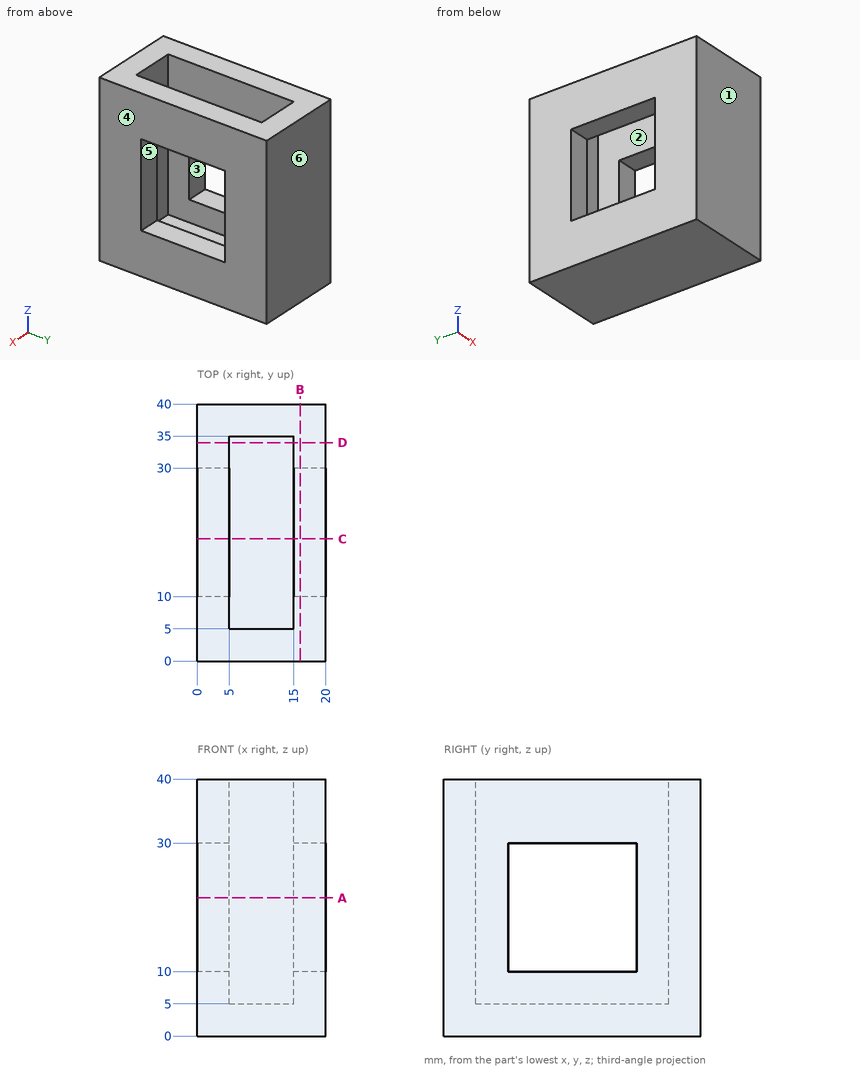
Design review of the part shown in the three views and the two pictorial views. Dimensions are in mm from the part's minimum x, y and z. A direction names the side the tool comes from. Round coordinates to 2 decimals unless told otherwise and drop trailing zeros. Order: outer loops, then holes, each group sorted by start corner. A loop starts at its lowest first (then second) coordinate and runs counter-clockwise, first axis right, second up. Notation, with made-up numbers: M 56.5,43.5 L 94.5,43.5 A24 ccw 94.5,68.5 Z; hole C 29.5,37 d1. An arc over 180 degrees is marked long. Put each result on its own line as item: value.
Q1. Consider section D-D (y = 34). State the section outline as (x, z) points, and give its area (3 significant figures).
Reported:
outline: M 0,0 L 20,0 L 20,40 L 15,40 L 15,5 L 5,5 L 5,40 L 0,40 Z
area: 450 mm²
Q2. Insertion check: pin 1 Ø1 at (x, y) = (9.5, 18.5) entering from +Z. The pin has a flat end and moves straight along its axis. Give the tip position at first contact, or say it passes through.
Reported:
pin 1: z = 5
Q3. Consider section A-A (z = 21.5). State the section outline as (x, y) points, and give its area (3 significant figures).
Reported:
outline: M 0,0 L 20,0 L 20,10 L 15,10 L 15,5 L 5,5 L 5,10 L 0,10 Z; M 0,30 L 5,30 L 5,35 L 15,35 L 15,30 L 20,30 L 20,40 L 0,40 Z
area: 300 mm²
Q4. Consider section B-B (x = 16). State the section outline as (y, z) points.
Reported:
outline: M 0,0 L 40,0 L 40,40 L 0,40 Z; hole M 10,10 L 30,10 L 30,30 L 10,30 Z
Q5. To check wall thickness, follow line 1 (Z direction, x = 1.5, y = 22.5); line 2 (Y direction, x = 9.5, z = 20.5); line 3 (X direction, y = 34, z = 9). State the ranges of each line that lie inside material, in increasing order.
Reported:
line 1: 0 to 10, 30 to 40
line 2: 0 to 5, 35 to 40
line 3: 0 to 5, 15 to 20
Q6. Machinability: for the marked faces 1, 2 and 3, which of the approach directions +Z, -Z, +X, -X, +Y, -Y give a long, thin tool a straight path to every point of the face, cutting with its end or side? Answer none if there is none.
Reported:
face 1: +Z, -Z, +X, -X, -Y
face 2: +Z
face 3: +X, -X
Q7. Consider section C-C (y = 19). State the section outline as (x, z) points, and give its area (3 significant figures).
Reported:
outline: M 0,0 L 20,0 L 20,10 L 15,10 L 15,5 L 5,5 L 5,10 L 0,10 Z; M 0,30 L 5,30 L 5,40 L 0,40 Z; M 15,30 L 20,30 L 20,40 L 15,40 Z
area: 250 mm²
Q8. Draft analysis for pull direction Y (two halves, no side actions). For the marked faces 4, 5 and 6, state which applies: released by +Y, released by -Y, zero draft, split by the parting line, or undercut.
Reported:
face 4: zero draft
face 5: undercut
face 6: released by +Y
